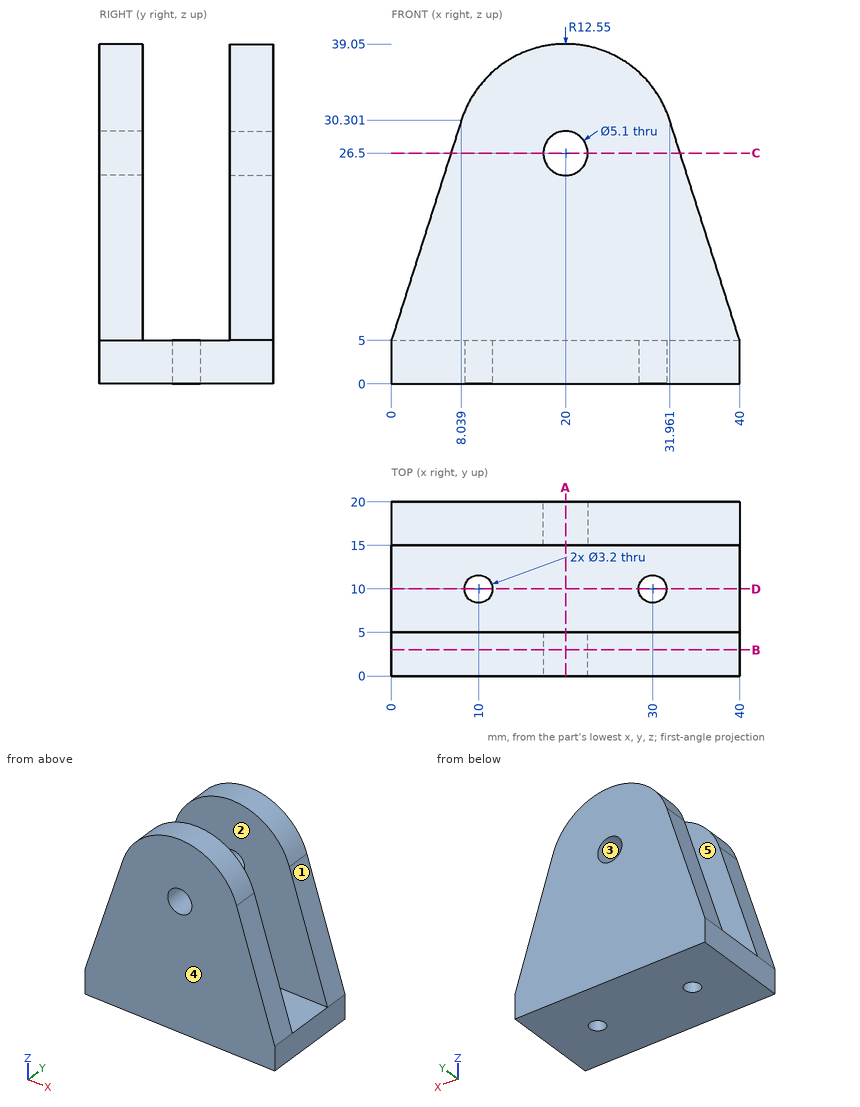
Print and shaded views of the part. All mm, measured from the part's lowest x, y and z. A direction names the side the tool comes from. Coordinates: 2 decimals unless noted, no trailing zeros. Loops run counter-clockwise (first coordinate to the right, second up) from the corner with the lowest first, then second, coordinate; pieces in that order, holes last. Notation, with made-up numbers: (58.25, 56) -> (83.25, 56) arc R24 ccw to (83.25, 67) -> close; hole circle Ø10 at (20.25, 87). An arc over 180 degrees is marked (long way). Use a Markdown table: item, result. Add a question column.
Item 1: Pull direction Y, two halves, no side cores. Call the marked faces 3, 4 and 5: +Y half, -Y half, draft (parallel to the pull), parting line (faces both ways), or undercut.
Item 2: Flat gauge pins, fed straight in: P1, Ø1, axis at x = 13, y = 5, coming from the -Z side; P2, Ø5, axis at x = 10, y = 10, coming from the +Z side; P3, Ø1.9, axis at x = 30, y = 10, coming from the +Z side (3 decimals); P4, Ø12, axis at x = 10.5, y = 2.5, coming from the +Z side. Where does each tip first touch, or does it go through?
Item 3: Band-saw the part on B-B on y = 3. Write the cut outline in (x, z).
Item 4: Band-saw the part on D-D on y = 10. Write the cut outline in (x, z), plus the area to 3 significant figures.
Item 5: Which spindle directions (+Z, -Z, +X, -X, +Y, -Y) get a long thin tool onto all of the face, cutting with end or side? Do the marked faces 1 and 2. Say none if no direction does.
Item 6: Band-saw the part on C-C on z = 26.5. Write the cut outline in (x, y), plus the area to 3 significant figures.
Item 7: Band-saw the part on A-A on x = 20. Write the cut outline in (y, z).
Item 8: Probe probe 1 along Y at (x, z) = (23, 21); probe 2 along Y at (x, z) = (10, 3.1); probe 3 along Z at (x, y) = (20, 3.7). List the from-to ranges inside material, lowest first.
Geometry says:
| question | item | result |
|---|---|---|
| 1 | face 3 | draft |
| 1 | face 4 | -Y half |
| 1 | face 5 | undercut |
| 2 | P1 | z = 0 |
| 2 | P2 | z = 5 |
| 2 | P3 | through |
| 2 | P4 | z = 38.55 |
| 3 | outline | (0, 0) -> (40, 0) -> (40, 5) -> (31.96, 30.3) arc R12.55 ccw to (8.04, 30.3) -> (0, 5) -> close; hole circle Ø5.1 at (20, 26.5) |
| 4 | outline | (0, 0) -> (8.4, 0) -> (8.4, 5) -> (0, 5) -> close; (11.6, 0) -> (28.4, 0) -> (28.4, 5) -> (11.6, 5) -> close; (31.6, 0) -> (40, 0) -> (40, 5) -> (31.6, 5) -> close |
| 4 | area | 168 mm² |
| 5 | face 1 | +Z, +X, +Y, -Y |
| 5 | face 2 | +Z, +X, -X |
| 6 | outline | (6.83, 0) -> (17.45, 0) -> (17.45, 5) -> (6.83, 5) -> close; (6.83, 15) -> (17.45, 15) -> (17.45, 20) -> (6.83, 20) -> close; (22.55, 0) -> (33.17, 0) -> (33.17, 5) -> (22.55, 5) -> close; (22.55, 15) -> (33.17, 15) -> (33.17, 20) -> (22.55, 20) -> close |
| 6 | area | 212 mm² |
| 7 | outline | (0, 0) -> (20, 0) -> (20, 23.95) -> (15, 23.95) -> (15, 5) -> (5, 5) -> (5, 23.95) -> (0, 23.95) -> close; (0, 29.05) -> (5, 29.05) -> (5, 39.05) -> (0, 39.05) -> close; (15, 29.05) -> (20, 29.05) -> (20, 39.05) -> (15, 39.05) -> close |
| 8 | probe 1 | 0 to 5, 15 to 20 |
| 8 | probe 2 | 0 to 8.4, 11.6 to 20 |
| 8 | probe 3 | 0 to 23.95, 29.05 to 39.05 |
